CAD build for the part. Positions are in the model's coordinates, mm. Round coordinates to 2 decimals unless told otherwise and drop trailing zeros. Loops run counter-clockwise (first coordinate to the right, second up) from the corner with the lowest first, then second, coordinate; pieces in that order, holes last.
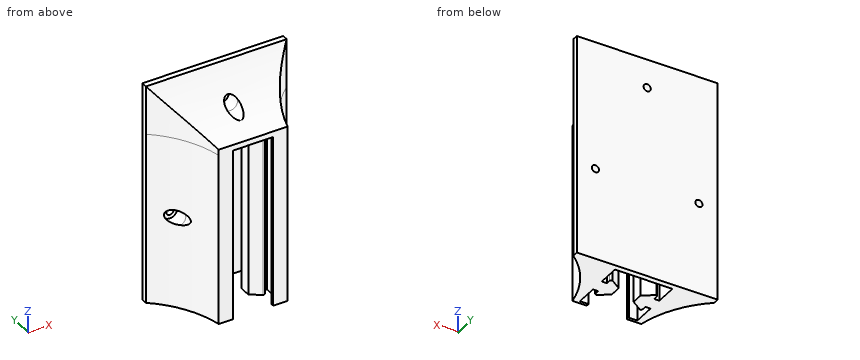
```python
from build123d import *

# Parameters (mm, degrees)
BOSS_EXTRUDE1_DEPTH                  = 38.1
BOSS_EXTRUDE3_DEPTH                  = 76.2
BOSS_EXTRUDE2_REACH                  = 53.498
BOSS_EXTRUDE2_END_RADIUS             = 44.45
BOSS_EXTRUDE2_DIRECTION_2_REACH      = 53.498
BOSS_EXTRUDE2_DIRECTION_2_END_RADIUS = 44.45
CUT_EXTRUDE3_DEPTH                   = 86.067352916
CUT_EXTRUDE1_REACH                   = 71.308
SKETCH4_R                            = 3.175
CUT_EXTRUDE1_DIRECTION_2_DEPTH       = 6.35
CUT_EXTRUDE2_REACH                   = 73.089
SKETCH5_R                            = 1.5875
LPATTERN1_COUNT                      = 2
LPATTERN1_PITCH                      = 44.45
LPATTERN1_COUNT_DIR2                 = 2
LPATTERN1_PITCH_DIR2                 = 22.86
MIRROR1_COPY_1_REACH                 = 71.308
MIRROR1_COPY_1_SKETCH_R              = 3.175
MIRROR1_COPY_2_SKETCH_R              = 3.175
MIRROR1_COPY_2_DEPTH                 = 6.35
MIRROR1_COPY_3_REACH                 = 73.089
MIRROR1_COPY_3_SKETCH_R              = 1.5875


with BuildPart() as part:
    # Sketch1 → Boss-Extrude1 (new, symmetric)
    with BuildSketch(Plane.XY):
        with BuildLine():
            Line((12.7, 12.7), (-12.7, 12.7))
            Line((-12.7, 12.7), (-12.7, 3.175))
            Line((-12.7, 3.175), (-10.414, 3.175))
            Line((-10.414, 3.175), (-10.414, 5.148491853))
            ThreePointArc((-10.414, 5.148491853), (-10.075709883, 5.709908138), (-9.421281116, 5.673146216))
            Line((-9.421281116, 5.673146216), (-4.826, 2.54))
            Line((-4.826, 2.54), (-4.826, -2.54))
            Line((-4.826, -2.54), (-9.421281116, -5.673146216))
            ThreePointArc((-9.421281116, -5.673146216), (-10.075709883, -5.709908138), (-10.414, -5.148491853))
            Line((-10.414, -5.148491853), (-10.414, -3.175))
            Line((-10.414, -3.175), (-12.7, -3.175))
            Line((-12.7, -3.175), (-12.7, -12.7))
            Line((-12.7, -12.7), (-8.89, -12.7))
            Line((-8.89, -12.7), (-8.89, -13.97))
            Line((-8.89, -13.97), (-15.24, -13.97))
            Line((-15.24, -13.97), (-15.24, 15.24))
            Line((-15.24, 15.24), (15.24, 15.24))
            Line((15.24, 15.24), (15.24, -13.97))
            Line((15.24, -13.97), (8.89, -13.97))
            Line((8.89, -13.97), (8.89, -12.7))
            Line((8.89, -12.7), (12.7, -12.7))
            Line((12.7, -12.7), (12.7, -3.175))
            Line((12.7, -3.175), (10.414, -3.175))
            Line((10.414, -3.175), (10.414, -5.148491853))
            ThreePointArc((10.414, -5.148491853), (10.075709883, -5.709908138), (9.421281116, -5.673146216))
            Line((9.421281116, -5.673146216), (4.826, -2.54))
            Line((4.826, -2.54), (4.826, 2.54))
            Line((4.826, 2.54), (9.421281116, 5.673146216))
            ThreePointArc((9.421281116, 5.673146216), (10.075709883, 5.709908138), (10.414, 5.148491853))
            Line((10.414, 5.148491853), (10.414, 3.175))
            Line((10.414, 3.175), (12.7, 3.175))
            Line((12.7, 3.175), (12.7, 12.7))
        make_face()
    extrude(amount=BOSS_EXTRUDE1_DEPTH, both=True)

    # Sketch6 → Boss-Extrude3 (add)
    with BuildSketch(Plane(origin=(0, 0, -38.1), x_dir=(-1, 0, 0), z_dir=(0, 0, -1))):
        with BuildLine():
            Line((-15.24, 15.24), (-31.115, 15.24))
            Line((-31.115, 15.24), (-31.115, 12.7))
            ThreePointArc((-31.115, 12.7), (-20.774098647, 0.795596044), (-15.24, -13.97))
            Line((-15.24, -13.97), (-15.24, 15.24))
        make_face()
        with BuildLine():
            Line((15.24, 15.24), (31.115, 15.24))
            Line((31.115, 15.24), (31.115, 12.7))
            ThreePointArc((31.115, 12.7), (20.774098647, 0.795596044), (15.24, -13.97))
            Line((15.24, -13.97), (15.24, 15.24))
        make_face()
    extrude(amount=-BOSS_EXTRUDE3_DEPTH)

    # Boss-Extrude2: up to this cylinder (the profile starts outside it)
    boss_extrude2_end = Plane(origin=(58.969667359, -21.939861523, 45.16983), z_dir=(0, 0, -1)) * Cylinder(BOSS_EXTRUDE2_END_RADIUS, 196.896, mode=Mode.PRIVATE)
    # Sketch3 → Boss-Extrude2 (add, up to the surface)
    with BuildSketch(Plane(origin=(0, 0, 0), x_dir=(0, 0, -1), z_dir=(1, 0, 0)), mode=Mode.PRIVATE) as boss_extrude2_sk1:
        with BuildLine():
            Line((-59.69, 15.24), (-59.69, 12.7))
            ThreePointArc((-59.69, 12.7), (-47.617150174, 1.184892733), (-40.64, -13.97))
            Line((-40.64, -13.97), (-38.1, -13.97))
            Line((-38.1, -13.97), (-38.1, 15.24))
            Line((-38.1, 15.24), (-59.69, 15.24))
        make_face()
    boss_extrude2_tool1 = extrude(boss_extrude2_sk1.sketch, amount=BOSS_EXTRUDE2_REACH, mode=Mode.PRIVATE) - boss_extrude2_end
    add(boss_extrude2_tool1.solids().sort_by_distance((0, 5.474065, 45.16983))[0])

    # Boss-Extrude2 direction 2: up to this cylinder (the profile starts outside it)
    boss_extrude2_direction_2_end = Plane(origin=(-58.969667359, -21.939861523, 45.16983), z_dir=(0, 0, -1)) * Cylinder(BOSS_EXTRUDE2_DIRECTION_2_END_RADIUS, 196.896, mode=Mode.PRIVATE)
    # Sketch3 → Boss-Extrude2 direction 2 (add, up to the surface)
    with BuildSketch(Plane(origin=(0, 0, 0), x_dir=(0, 0, -1), z_dir=(1, 0, 0)), mode=Mode.PRIVATE) as boss_extrude2_direction_2_sk1:
        with BuildLine():
            Line((-59.69, 15.24), (-59.69, 12.7))
            ThreePointArc((-59.69, 12.7), (-47.617150174, 1.184892733), (-40.64, -13.97))
            Line((-40.64, -13.97), (-38.1, -13.97))
            Line((-38.1, -13.97), (-38.1, 15.24))
            Line((-38.1, 15.24), (-59.69, 15.24))
        make_face()
    boss_extrude2_direction_2_tool1 = extrude(boss_extrude2_direction_2_sk1.sketch, amount=-BOSS_EXTRUDE2_DIRECTION_2_REACH, mode=Mode.PRIVATE) - boss_extrude2_direction_2_end
    add(boss_extrude2_direction_2_tool1.solids().sort_by_distance((0, 5.474065, 45.16983))[0])

    # Sketch7 → Cut-Extrude3 (cut, through all)
    with BuildSketch(Plane(origin=(0, 0, 38.1), x_dir=(-1, 0, 0), z_dir=(0, 0, -1))):
        with BuildLine():
            Line((34.608624747, 15.24), (31.115, 15.24))
            Line((31.115, 15.24), (31.115, 12.7))
            ThreePointArc((31.115, 12.7), (32.830941454, 14.012461185), (34.608624747, 15.24))
        make_face()
        with BuildLine():
            Line((-31.115, 12.7), (-31.115, 15.24))
            Line((-31.115, 15.24), (-34.608624747, 15.24))
            ThreePointArc((-34.608624747, 15.24), (-32.830941454, 14.012461185), (-31.115, 12.7))
        make_face()
    extrude(amount=-CUT_EXTRUDE3_DEPTH, mode=Mode.SUBTRACT)

    # Sketch4 → Cut-Extrude1 (cut, up to next)
    with BuildSketch(Plane(origin=(0, 2.54, 0), x_dir=(1, 0, 0), z_dir=(0, 1, 0)), mode=Mode.PRIVATE) as cut_extrude1_sk1:
        with Locations(Location((0, -46.99, 0), (0, 0, 90))):
            Circle(SKETCH4_R)
    cut_extrude1_tool1 = extrude(cut_extrude1_sk1.sketch, amount=-CUT_EXTRUDE1_REACH, mode=Mode.PRIVATE) & part.part
    cut_extrude1 = cut_extrude1_tool1.solids().sort_by_distance((0, 2.54, 46.99))[0]
    add(cut_extrude1, mode=Mode.SUBTRACT)

    # Sketch4 → Cut-Extrude1 direction 2 (cut)
    with BuildSketch(Plane(origin=(0, 2.54, 0), x_dir=(1, 0, 0), z_dir=(0, 1, 0))):
        with Locations(Location((0, -46.99, 0), (0, 0, 90))):
            Circle(SKETCH4_R)
    cut_extrude1_direction_2 = extrude(amount=CUT_EXTRUDE1_DIRECTION_2_DEPTH, mode=Mode.SUBTRACT)

    # Sketch5 → Cut-Extrude2 (cut, up to next)
    with BuildSketch(Plane.XZ.offset(-8.89), mode=Mode.PRIVATE) as cut_extrude2_sk1:
        with Locations(Location((0, 46.99, 0), (0, 0, 270))):
            Circle(SKETCH5_R)
    cut_extrude2_tool1 = extrude(cut_extrude2_sk1.sketch, amount=-CUT_EXTRUDE2_REACH, mode=Mode.PRIVATE) & part.part
    cut_extrude2 = cut_extrude2_tool1.solids().sort_by_distance((0, 8.89, 46.99))[0]
    add(cut_extrude2, mode=Mode.SUBTRACT)

    # LPattern1: Cut-Extrude1, Cut-Extrude1 direction 2, Cut-Extrude2; each copy of Cut-Extrude1, Cut-Extrude2 runs up to whatever stops it at its own place
    lpattern1_before = part.part  # the part as the pattern finds it: every copy runs up to it
    lpattern1_cut_extrude1_long = extrude(cut_extrude1_sk1.sketch, amount=-CUT_EXTRUDE1_REACH, mode=Mode.PRIVATE)
    lpattern1_cut_extrude1_tool1 = lpattern1_cut_extrude1_long.moved(Location(Vector(0, 0, -1) * (1 * LPATTERN1_PITCH) + Vector(1, 0, 0) * (1 * LPATTERN1_PITCH_DIR2))) & lpattern1_before
    add(lpattern1_cut_extrude1_tool1.solids().sort_by_distance((22.86, 2.54, 2.54))[0], mode=Mode.SUBTRACT)
    add(cut_extrude1_direction_2.moved(Location(Vector(0, 0, -1) * (1 * LPATTERN1_PITCH) + Vector(1, 0, 0) * (1 * LPATTERN1_PITCH_DIR2))), mode=Mode.SUBTRACT)
    lpattern1_cut_extrude2_long = extrude(cut_extrude2_sk1.sketch, amount=-CUT_EXTRUDE2_REACH, mode=Mode.PRIVATE)
    lpattern1_cut_extrude2_tool1 = lpattern1_cut_extrude2_long.moved(Location(Vector(0, 0, -1) * (1 * LPATTERN1_PITCH) + Vector(1, 0, 0) * (1 * LPATTERN1_PITCH_DIR2))) & lpattern1_before
    add(lpattern1_cut_extrude2_tool1.solids().sort_by_distance((22.86, 8.89, 2.54))[0], mode=Mode.SUBTRACT)

    # Mirror1 copy 1 sketch → Mirror1 copy 1 (cut, up to next)
    with BuildSketch(Plane(origin=(-22.86, 2.54, -44.45), x_dir=(-1, 0, 0), z_dir=(0, 1, 0)), mode=Mode.PRIVATE) as mirror1_copy_1_sk1:
        with Locations((0, 46.99)):
            Circle(MIRROR1_COPY_1_SKETCH_R)
    mirror1_copy_1_tool1 = extrude(mirror1_copy_1_sk1.sketch, amount=-MIRROR1_COPY_1_REACH, mode=Mode.PRIVATE) & part.part
    add(mirror1_copy_1_tool1.solids().sort_by_distance((-22.86, 2.54, 2.54))[0], mode=Mode.SUBTRACT)

    # Mirror1 copy 2 sketch → Mirror1 copy 2 (cut)
    with BuildSketch(Plane(origin=(-22.86, 2.54, -44.45), x_dir=(-1, 0, 0), z_dir=(0, 1, 0))):
        with Locations((0, 46.99)):
            Circle(MIRROR1_COPY_2_SKETCH_R)
    extrude(amount=MIRROR1_COPY_2_DEPTH, mode=Mode.SUBTRACT)

    # Mirror1 copy 3 sketch → Mirror1 copy 3 (cut, up to next)
    with BuildSketch(Plane(origin=(-22.86, 8.89, -44.45), x_dir=(-1, 0, 0), z_dir=(0, -1, 0)), mode=Mode.PRIVATE) as mirror1_copy_3_sk1:
        with Locations((0, -46.99)):
            Circle(MIRROR1_COPY_3_SKETCH_R)
    mirror1_copy_3_tool1 = extrude(mirror1_copy_3_sk1.sketch, amount=-MIRROR1_COPY_3_REACH, mode=Mode.PRIVATE) & part.part
    add(mirror1_copy_3_tool1.solids().sort_by_distance((-22.86, 8.89, 2.54))[0], mode=Mode.SUBTRACT)


solid = part.part
```
Item 1: Probe line 1 (X direction, y = 13.25, z = 2.54) (1 decimal); line 2 (Y direction, x = -12, z = -17.5) (3 decimals); line 3 (X direction, y = 5, z = 2.54) (3 decimals). List the from-to ranges inside material, lowest first.
Answers follow:
line 1: x = -31.1 to -24.4, -21.3 to 21.3, 24.4 to 31.1
line 2: y = -13.97 to -12.7, -3.175 to 3.175, 12.7 to 15.24
line 3: x = -19.685 to -12.7, -10.414 to -8.434, 8.434 to 10.414, 12.7 to 19.685
Item 2: Cut at D-D, the plane y = 1.5. Give the cut face in (x, z) (3 decimals), plus the area to 3 significant figures.
Answers follow:
outline: (-21.202, -38.1) - (-4.826, -38.1) - (-4.826, 38.1) - (4.826, 38.1) - (4.826, -38.1) - (21.202, -38.1) - (21.202, -0.168) arc R3.175 cw to (21.202, 5.248) - (21.202, 47.844) - (3.058, 47.844) arc R3.175 cw (long way) to (-3.058, 47.844) - (-21.202, 47.844) - (-21.202, 5.248) arc R3.175 cw to (-21.202, -0.168) - close
area: 2,880 mm2
Item 3: Flat gauge pins, fed straight in: P1, Ø5, axis at x = -22.86, z = 2.54, coming from the -Y side; P2, Ø6, axis at y = -4, z = -12, coming from the -X side; P3, Ø8, axis at x = 23.5, y = -4.5, coming from the -Z side; P4, Ø1, axis at y = -6, z = 41.5, coming from the -X side. Where does each tip first touch, or does it go through?
Answers follow:
P1: stops at y = 8.89
P2: stops at x = -19.76
P3: passes through
P4: stops at x = -17.67
